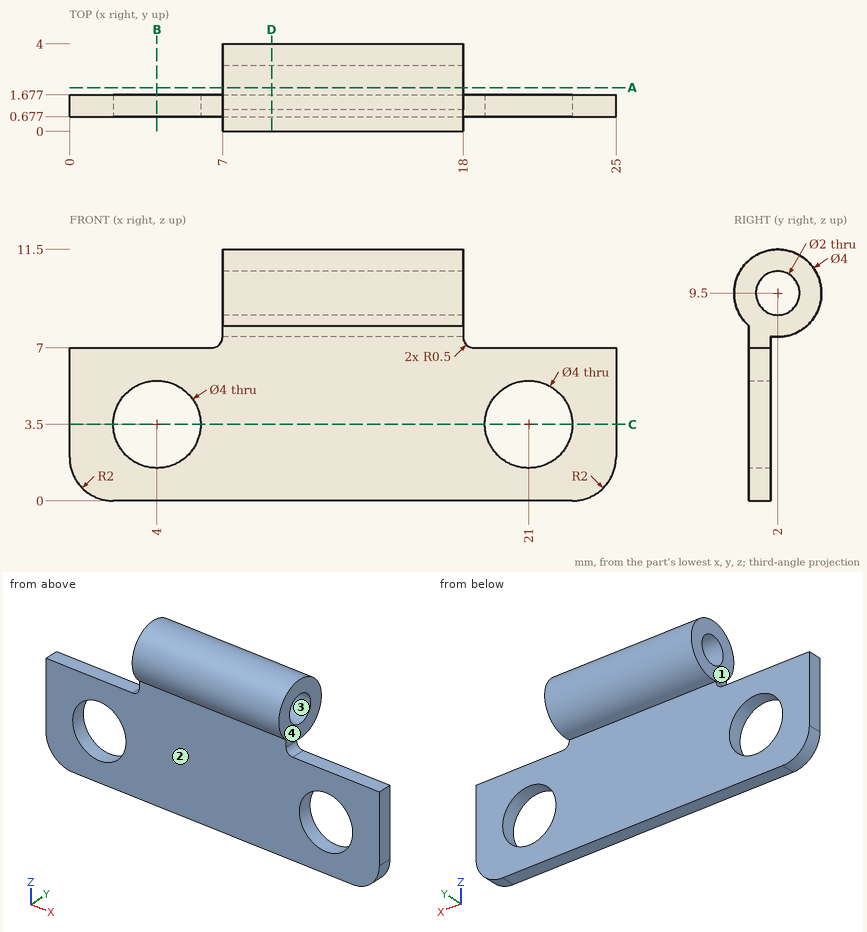
Design review of the part shown in the three views and the two pictorial views. Dimensions are in mm from the part's minimum x, y and z. A direction names the side the tool comes from. Round coordinates to 2 decimals unless told otherwise and drop trailing zeros. Write each loop counter-clockwise with the first axis right and the second up, starting at its lowest first coordinate (ties: lowest second). Pieces come first, ordered by that corner, then holes.
1) Insertion check: pin 1 Ø4.5 at (x, z) = (21, 3.5) entering from +Y; pin 2 Ø4 at (x, z) = (13, 6) entering from +Y; pin 3 Ø5 at (x, z) = (4, 3.5) entering from -Y. Each pin has a flat end and moves straight along its axis. Give the tip position at first contact, or say it passes through.
Answer below:
pin 1: stops at y = 1.68
pin 2: stops at y = 3.32
pin 3: stops at y = 0.68
2) Machinability: for the marked faces 1, 2, 3 and 4, which of the approach directions +Z, -Z, +X, -X, +Y, -Y give a long, thin tool a straight path to every point of the face, cutting with its end or side? Answer none if there is none.
Answer below:
face 1: +Z, -X, +Y, -Y
face 2: -Z, +X, -X, -Y
face 3: +X, -X
face 4: +Z, +X, +Y, -Y
3) For line 1 along X through (y, z) = (1.15, 3.5); line 2 along X through (y, z) = (0.8, 4.25); line 3 along Y through (x, z) = (9.5, 9.5), list the stretches that pass through material, from the lowest coordinate up.
Answer below:
line 1: x = 0 to 2, 6 to 19, 23 to 25
line 2: x = 0 to 2.15, 5.85 to 19.15, 22.85 to 25
line 3: y = 0 to 1, 3 to 4
4) Take a section at D-D on x = 9.25. Give the boundary of the cut face in (y, z).
Answer below:
outline: (0.68, 0) - (1.68, 0) - (1.68, 7.53) arc R2 ccw (long way) to (0.68, 8) - close; hole circle Ø2 at (2, 9.5)
5) Take a section at A-A on y = 2. Give the boundary of the cut face in (x, z).
Answer below:
outline: (7, 7.5) - (18, 7.5) - (18, 8.5) - (7, 8.5) - close; (7, 10.5) - (18, 10.5) - (18, 11.5) - (7, 11.5) - close
6) Take a section at C-C on z = 3.5. Give the boundary of the cut face in (x, y), then the cut area to 3 significant figures.
Answer below:
outline: (0, 0.68) - (2, 0.68) - (2, 1.68) - (0, 1.68) - close; (6, 0.68) - (19, 0.68) - (19, 1.68) - (6, 1.68) - close; (23, 0.68) - (25, 0.68) - (25, 1.68) - (23, 1.68) - close
area: 17.0 mm2
7) Take a section at B-B on x = 4. Give the boundary of the cut face in (y, z).
Answer below:
outline: (0.68, 0) - (1.68, 0) - (1.68, 1.5) - (0.68, 1.5) - close; (0.68, 5.5) - (1.68, 5.5) - (1.68, 7) - (0.68, 7) - close
